```python
from build123d import *

# Parameters (mm, degrees)
SKETCH1_W           = 20
SKETCH1_H           = 7
BOSS_EXTRUDE1_DEPTH = 0.3
SKETCH2_W           = 13
SKETCH2_H           = 7
BOSS_EXTRUDE2_DEPTH = 8.4
CUT_EXTRUDE5_REACH  = 2.3
SKETCH3_R           = 1.25
SKETCH4_R           = 0.4
BOSS_EXTRUDE3_DEPTH = 4.8


with BuildPart() as part:
    # Sketch1 → Boss-Extrude1 (new body)
    with BuildSketch(Plane(origin=(0, 0, 0), x_dir=(1, 0, 0), z_dir=(0, 1, 0))):
        Rectangle(SKETCH1_W, SKETCH1_H)
    extrude(amount=BOSS_EXTRUDE1_DEPTH)

    # Sketch2 → Boss-Extrude2 (add)
    with BuildSketch(Plane(origin=(0, 0.3, 0), x_dir=(1, 0, 0), z_dir=(0, 1, 0))):
        Rectangle(SKETCH2_W, SKETCH2_H)
    extrude(amount=BOSS_EXTRUDE2_DEPTH)

    # Sketch3 → Cut-Extrude5 (cut, up to next)
    with BuildSketch(Plane(origin=(0, 0.3, 0), x_dir=(1, 0, 0), z_dir=(0, 1, 0)), mode=Mode.PRIVATE) as cut_extrude5_sk1:
        with Locations((-8.74, 0)):
            Circle(SKETCH3_R)
    cut_extrude5_tool1 = extrude(cut_extrude5_sk1.sketch, amount=-CUT_EXTRUDE5_REACH, mode=Mode.PRIVATE) & part.part
    add(cut_extrude5_tool1.solids().sort_by_distance((-8.74, 0.3, 0))[0], mode=Mode.SUBTRACT)
    # Sketch3 → Cut-Extrude5 (cut, up to next)
    with BuildSketch(Plane(origin=(0, 0.3, 0), x_dir=(1, 0, 0), z_dir=(0, 1, 0)), mode=Mode.PRIVATE) as cut_extrude5_sk2:
        with Locations((8.74, 0)):
            Circle(SKETCH3_R)
    cut_extrude5_tool2 = extrude(cut_extrude5_sk2.sketch, amount=-CUT_EXTRUDE5_REACH, mode=Mode.PRIVATE) & part.part
    add(cut_extrude5_tool2.solids().sort_by_distance((8.74, 0.3, 0))[0], mode=Mode.SUBTRACT)

    # Sketch4 → Boss-Extrude3 (add)
    with BuildSketch(Plane(origin=(0, 8.7, 0), x_dir=(1, 0, 0), z_dir=(0, 1, 0))):
        with Locations((-4.6, 0)):
            Circle(SKETCH4_R)
        Circle(SKETCH4_R)
        with Locations((4.6, 0)):
            Circle(SKETCH4_R)
    extrude(amount=BOSS_EXTRUDE3_DEPTH)


solid = part.part
```
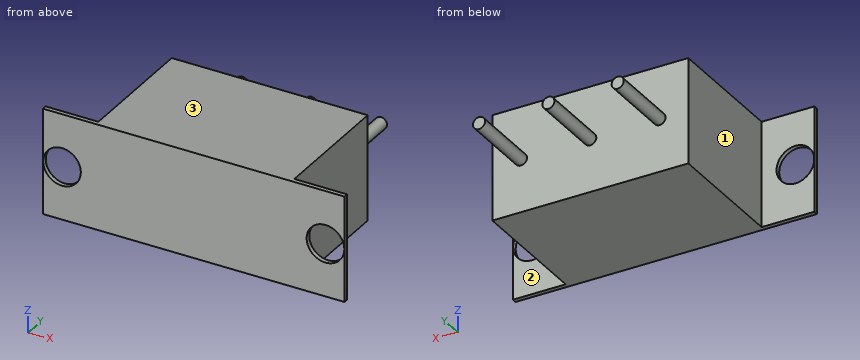
Model file for the job. Use its own axes, mm. Face numbers are marked on the shaded views. A direction names the side the tool comes from. Coordinates: 2 decimals unless noted, no trailing zeros. Order: outer loops, then holes, each group sorted by start corner. A loop starts at its lowest first (then second) coordinate and runs counter-clockwise, first axis right, second up. Notation, with made-up numbers: (30.25, 78.25) - (36.25, 78.25) arc R12 ccw to (36.25, 97.25) - close; hole circle Ø8 at (-13.75, 75.5). An arc over 180 degrees is marked (long way). Return JSON: item names as keys, results as strings. Group by question number.
1) Tool access for the marked faces 1, 2 and 3: list every direction of +Z, -Z, +X, -X, +Y, -Y with a clear straight run to the whole face (end or side of a thin tool).
2) Saw through at C-C, the plane x = 4.6. Write the cut outline in (y, z).
3) Flat gauge pins, fed straight in: P1, Ø1, axis at x = -7.5, z = -0.5, coming from the +Y side; P2, Ø3, axis at x = 8, z = -1.5, coming from the -Y side; P3, Ø3, axis at y = 12, z = 3, coming from the +X side; P4, Ø2, axis at y = 7.5, z = 1, coming from the -X side. Where does each tip first touch, or does it go through?
4) Saw through at D-D, the plane y = 11.5. Write the cut outline in (x, z).
5) Saw through at A-A, the plane x = -8.74. Write the cut outline in (y, z), plus the area to 3 significant figures.
6) Probe line 1 (X direction, y = 1.5, z = 0); line 2 (Y direction, x = -3, z = -1.75). List the from-to ranges inside material, lowest first. Write a range as from..to.
7) Saw through at B-B, the plane z = 0. Count the separate pieces of the cut face and the enclosed holes in it, plus the area to 3 significant figures.
Values found:
{
 "1": {"face 1": "+Z, -Z, -X, +Y", "face 2": "+Z, -Z, +X, +Y", "face 3": "+Z, +X, -X, +Y, -Y"},
 "2": {"outline": "(0, -3.5) - (8.7, -3.5) - (8.7, -0.4) - (13.5, -0.4) - (13.5, 0.4) - (8.7, 0.4) - (8.7, 3.5) - (0, 3.5) - close"},
 "3": {"P1": "stops at y = 0.3", "P2": "stops at y = 0", "P3": "passes through", "P4": "stops at x = -6.5"},
 "4": {"outline": "circle Ø0.8 at (-4.6, 0); circle Ø0.8 at (0, 0); circle Ø0.8 at (4.6, 0)"},
 "5": {"outline": "(0, -3.5) - (0.3, -3.5) - (0.3, -1.25) - (0, -1.25) - close; (0, 1.25) - (0.3, 1.25) - (0.3, 3.5) - (0, 3.5) - close", "area": "1.35 mm²"},
 "6": {"line 1": "x = -6.5..6.5", "line 2": "y = 0..8.7"},
 "7": {"separate pieces": "3", "enclosed holes": "0", "area": "125 mm²"}
}
